Input: dimensioned drawing with shaded views. Units: mm. Origin: part minimum x, y, z. Coordinates: 2 decimals unless noted, no trailing zeros. Order: outer loops, then holes, each group sorted by start corner. A loop starts at its lowest first (then second) coordinate and runs counter-clockwise, first axis right, second up.
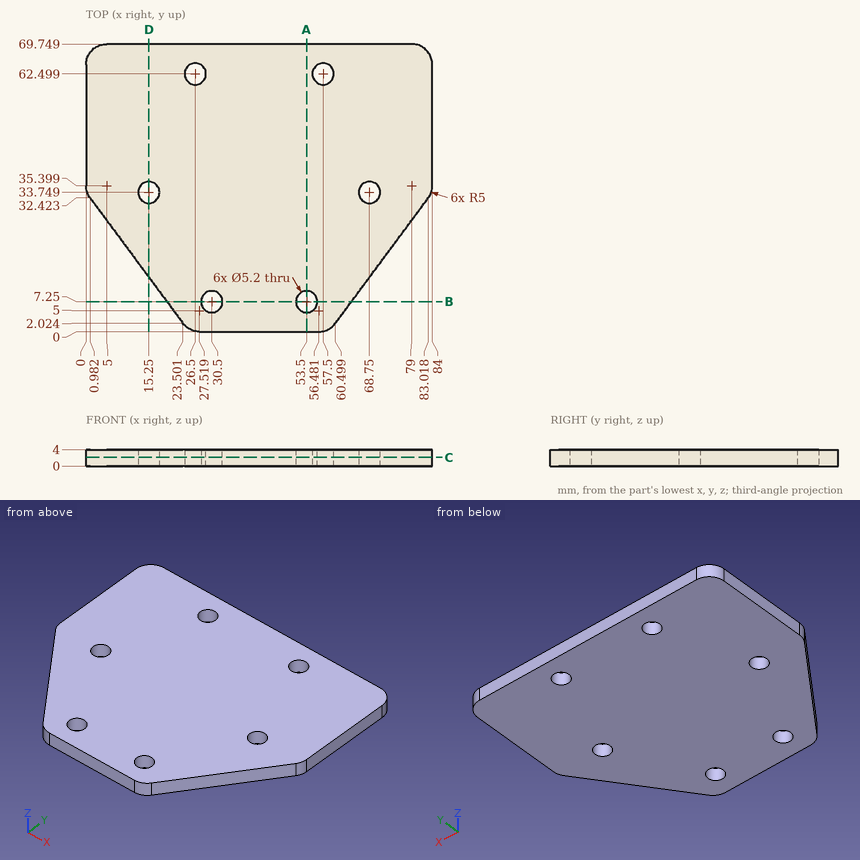
1. Section query D-D on x = 15.25. Return loops of the section in (y, z).
Findings:
outline: (13.16, 0) - (31.15, 0) - (31.15, 4) - (13.16, 4) - close; (36.35, 0) - (69.75, 0) - (69.75, 4) - (36.35, 4) - close
2. Ray query, line 1 (X direction, y = 63, z = 3); line 2 (Y direction, x = 53.5, z = 1); line 3 (X direction, y = 61, z = 1.1) (1 decimal). Return the intervals inside material, ascending.
Findings:
line 1: x = 0 to 23.95, 29.05 to 54.95, 60.05 to 84
line 2: y = 0 to 4.65, 9.85 to 69.75
line 3: x = 0 to 24.4, 28.6 to 55.4, 59.6 to 84
3. Section query C-C on z = 2.1. Return loops of the section in (x, y).
Findings:
outline: (0, 35.4) arc R5 ccw to (0.98, 32.42) - (23.5, 2.02) arc R5 ccw to (27.52, 0) - (56.48, 0) arc R5 ccw to (60.5, 2.02) - (83.02, 32.42) arc R5 ccw to (84, 35.4) - (84, 64.75) arc R5 ccw to (79, 69.75) - (5, 69.75) arc R5 ccw to (0, 64.75) - close; hole circle Ø5.2 at (15.25, 33.75); hole circle Ø5.2 at (26.5, 62.5); hole circle Ø5.2 at (30.5, 7.25); hole circle Ø5.2 at (53.5, 7.25); hole circle Ø5.2 at (57.5, 62.5); hole circle Ø5.2 at (68.75, 33.75)
4. Section query A-A on x = 53.5. Return loops of the section in (y, z), plus the area to 3 significant figures.
Findings:
outline: (0, 0) - (4.65, 0) - (4.65, 4) - (0, 4) - close; (9.85, 0) - (69.75, 0) - (69.75, 4) - (9.85, 4) - close
area: 258 mm2
5. Section query B-B on y = 7.25. Return loops of the section in (x, z).
Findings:
outline: (19.63, 0) - (27.9, 0) - (27.9, 4) - (19.63, 4) - close; (33.1, 0) - (50.9, 0) - (50.9, 4) - (33.1, 4) - close; (56.1, 0) - (64.37, 0) - (64.37, 4) - (56.1, 4) - close
6. Pin query (flat end, axial travel): P1, Ø1, axis at y = 22, z = 1, coming from the +X side; P2, Ø4, axis at x = 57.5, y = 62.5, coming from the -Z side; P3, Ø1, axis at x = 33, y = 45.5, coming from the -Z side. Return the tip coordinate at first contact, or that it passes through.
Findings:
P1: stops at x = 75.67
P2: passes through
P3: stops at z = 0
